CAD build for the part. Positions are in the model's coordinates, mm. Coordinates: 2 decimals unless noted, no trailing zeros. Order: outer loops, then holes, each group sorted by start corner. A loop starts at its lowest first (then second) coordinate and runs counter-clockwise, first axis right, second up. Notation, with made-up numbers: (20, 66) - (58, 66) arc R18 ccw to (58, 96) - close; hole circle Ø9 at (-27, -31). An arc over 180 degrees is marked (long way). Return JSON: item names as keys, results as strings.
Solid Edge part; units mm, degrees
sketch "Sketch1" plane through (0, 0, 0) normal (0, 0, 1) x (1, 0, 0)
  line L0 (-10, -10) -> (10, -10)
  line L1 (10, -10) -> (10, 10)
  line L2 (10, 10) -> (-10, 10)
  line L3 (-10, 10) -> (-10, -10)
extrude "Protrusion1" add sketch "Sketch1" along normal blind 41.1686
sketch "Sketch2" plane through (0, 10, 20.5843) normal (0, 1, 0) x (-1, 0, 0)
  line L0 (-10, -20.5843) -> (0, -3.2638)
extrude "ExtrudedCutout_1" cut sketch "Sketch2" along normal mid plane 135.5607 material side at (5.0433, 10, 8.6853)
pattern_circular "Pattern1" count 4 over 360 about axis through (0, 0, 0) along (0, 0, 1) of "ExtrudedCutout_1"
Item 1: Band-saw the part on B-B, the plane x = 7.75. List the corners of the cut face in (y, z), then the cut area to 3 significant figures.
Findings below:
{"outline": "(-10, 0) - (10, 0) - (7.75, 3.9) - (-7.75, 3.9) - close", "area": "69.2 mm²"}
Item 2: Drop flat-ended pins along their axis: P1, Ø1.5, axis at y = -5.5, z = 3.5, coming from the -X side; P2, Ø1, axis at y = 5, z = 8.5, coming from the -X side; P3, Ø1.5, axis at x = 4.5, y = 3, coming from the +Z side; P4, Ø12, axis at x = 0.5, y = 3.5, coming from the -Z side. Give the stop position or say it passes through.
Findings below:
{"P1": "stops at x = -8.41", "P2": "stops at x = -5.38", "P3": "stops at z = 10.83", "P4": "stops at z = 0"}
Item 3: Wall check: L1, parallel to Y at x = -1.5, z = 6; L2, parallel to Y at x = 5.25, z = 5; L3, parallel to X at y = -4.5, z = 1.25. Give the ranges that are in metal, low to high. Write a range as [from, to].
Findings below:
{"L1": "y = [-6.54, 6.54]", "L2": "y = [-7.11, 7.11]", "L3": "x = [-9.28, 9.28]"}
Item 4: Band-saw the part on A-A, the plane y = -1.25. List the corners of the cut face in (x, z), then the cut area to 3 significant figures.
Findings below:
{"outline": "(-10, 0) - (10, 0) - (1.25, 15.16) - (-1.25, 15.16) - close", "area": "170 mm²"}
